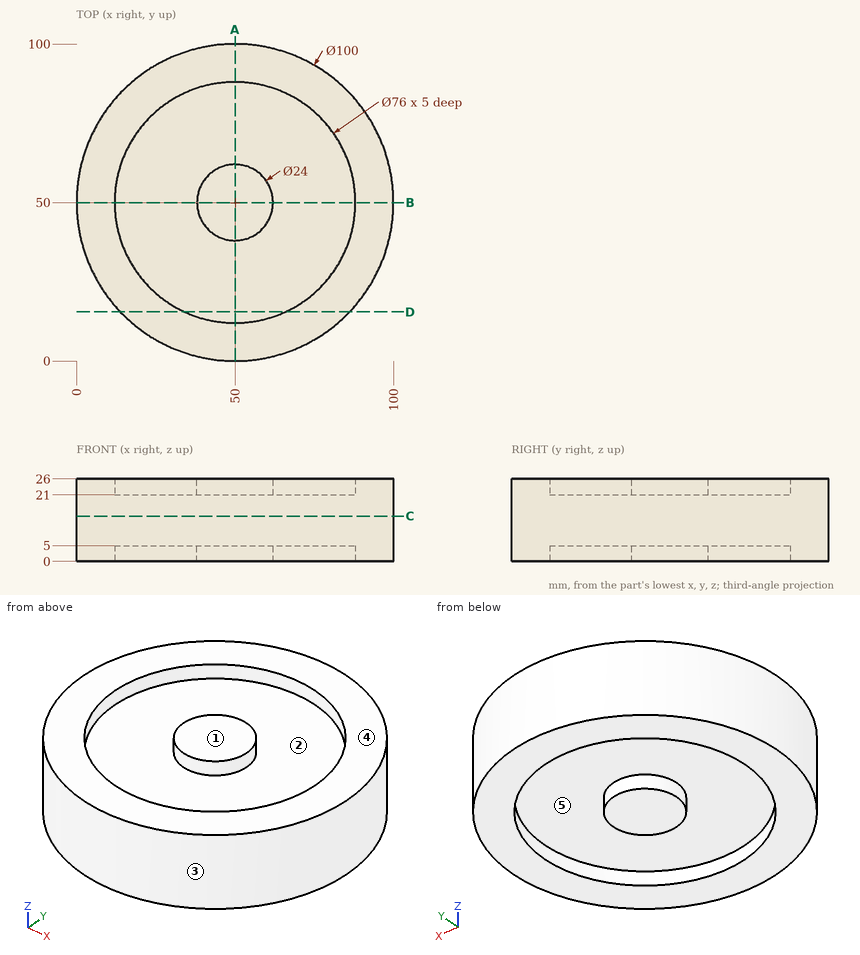
Job drawing, mm, ordinate dimensions from the low corner. One solid piece. A direction names the side the tool comes from. Give positions to 0.01 mm unless a question says otherwise; leave off trailing zeros. Write each loop counter-clockwise with the first axis right and the second up, starting at its lowest first coordinate (ties: lowest second). Pieces come first, ordered by that corner, then holes. Notation, with made-up numbers: M 0.5,-37.75 L 15.5,-37.75 A28 cw 15.5,-3.75 Z; hole C -27,31.5 d11. An arc over 180 degrees is marked long. Put each result on its own line as item: value. Start each with the question number.
(1) Band-saw the part on A-A, the plane x = 50. Write the cut outline in (y, z), and give its area (3 significant figures).
(2) Probe L1, parallel to Y at x = 50, z = 24.9; L2, parallel to X at y = 52.5, z = 24.75; L3, parallel to X at y = 47, z = 1.5. List the from-to ranges inside material, lowest first.
(3) Band-saw the part on D-D, the plane y = 15.5. Write the cut outline in (x, z).
(4) Mould opens along Y. For the marked faces 1, 2 and 3 say: +Y half, -Y half, draft (parallel to the pull), parting line (faces both ways), or undercut.
(5) Band-saw the part on C-C, the plane z = 14.25. Write the cut outline in (x, y), and give its area (3 significant figures).
(6) Flat gauge pins, fed straight in: pin 1 Ø2 at (y, z) = (59.5, 13.5) entering from -X; pin 2 Ø12 at (x, z) = (77.5, 20.5) entering from -Y; pin 3 Ø5 at (x, z) = (31.5, 8) entering from +Y. Where does each tip first touch, or does it go through?
(7) Which spindle directions (+Z, -Z, +X, -X, +Y, -Y) get a long thin tool onto all of the face, cutting with end or side? Do the marked faces 4 and 5. Say none if no direction does.
Response values:
1. outline: M 0,0 L 12,0 L 12,5 L 38,5 L 38,0 L 62,0 L 62,5 L 88,5 L 88,0 L 100,0 L 100,26 L 88,26 L 88,21 L 62,21 L 62,26 L 38,26 L 38,21 L 12,21 L 12,26 L 0,26 Z
1. area: 2,080 mm2
2. L1: y = 0 to 12, 38 to 62, 88 to 100
2. L2: x = 0.06 to 12.08, 38.26 to 61.74, 87.92 to 99.94
2. L3: x = 0.09 to 12.12, 38.38 to 61.62, 87.88 to 99.91
3. outline: M 13.81,0 L 34.07,0 L 34.07,5 L 65.93,5 L 65.93,0 L 86.19,0 L 86.19,26 L 65.93,26 L 65.93,21 L 34.07,21 L 34.07,26 L 13.81,26 Z
4. face 1: draft
4. face 2: undercut
4. face 3: parting line
5. outline: C 50,50 d100
5. area: 7,850 mm2
6. pin 1: stops at x = 0.73
6. pin 2: stops at y = 4.86
6. pin 3: stops at y = 97.37
7. face 4: +Z, +X, -X, +Y, -Y
7. face 5: -Z
